CAD build for the part. Positions are in the model's coordinates, mm. A direction names the side the tool comes from. Round coordinates to 2 decimals unless told otherwise and drop trailing zeros. Loops run counter-clockwise (first coordinate to the right, second up) from the corner with the lowest first, then second, coordinate; pieces in that order, holes last.
Autodesk Inventor part; units mm, degrees
ref_plane "Work Plane1" through (25, 0, 0) normal (1, 0, 0) x (0, 1, 0)
ref_plane "XZ Plane" through (0, 0, 0) normal (0, 1, 0) x (-1, 0, 0)
ref_plane "XY Plane" through (0, 0, 0) normal (0, 0, 1) x (1, 0, 0)
ref_plane "Work Plane1" through (25, 0, 0) normal (1, 0, 0) x (0, 1, 0)
sketch "Sketch1" plane through (0, 0, 0) normal (0, 0, 1) x (1, 0, 0)
  line L0 (0, 0) -> (50, 0)
  line L1 (50, 0) -> (50, 40)
  line L2 (50, 40) -> (0, 40)
  line L3 (0, 40) -> (0, 0)
  dimension "d0" = 50
  dimension "d1" = 40
extrude "Extrusion1" add sketch "Sketch1" along normal blind 30
sketch "Sketch3" plane through (50, 0, 0) normal (1, 0, 0) x (0, 0, -1)
  line L0 (0, 0) -> (-8, 40)
  line L1 (0, 40) -> (-30, 40)
  line L2 (0, 0) -> (40.7922, 0) construction
  arc A0 (0, 40) -> (-8, 40) centre (-4, 20) ccw
  line L3 (0, 0) -> (0, 40)
  line L4 (0, 40) -> (0, 0)
  dimension "d7" = 101.31
extrude "Extrusion3" cut sketch "Sketch3" against normal through all contours L0 L1 L3
sketch "Sketch4" plane through (0, 0, 30) normal (0, 0, 1) x (1, 0, 0)
  line L0 (0, 0) -> (50, 0) construction
  line L1 (25, 0) -> (25, 40) construction
  line L2 (50, 40) -> (0, 40) construction
  line L3 (0, 40) -> (0, 0) construction
  line L4 (0, 20) -> (50, 20) construction
  line L5 (50, 0) -> (50, 40) construction
  line L6 (17.5, 10) -> (17.5, 30)
  line L7 (32.5, 10) -> (32.5, 30)
  line L8 (12.5, 10) -> (12.5, 30)
  line L9 (37.5, 10) -> (37.5, 30)
  line L10 (12.5, 10) -> (17.5, 10)
  line L11 (32.5, 10) -> (37.5, 10)
  line L12 (12.5, 30) -> (17.5, 30)
  line L13 (32.5, 30) -> (37.5, 30)
  dimension "d12" = 7.5
  dimension "d13" = 7.5
  dimension "d14" = 5
  dimension "d15" = 20
  dimension "d16" = 5
  dimension "d17" = 20
  dimension "d18" = 10
  dimension "d19" = 10
extrude "Extrusion4" add sketch "Sketch4" along normal blind 22.5
fillet "Fillet1" radius 10 4 edges at (15, 10, 52.5) (15, 30, 52.5) (35, 10, 52.5) (35, 30, 52.5)
sketch "Sketch5" plane through (37.5, 10, 30) normal (1, 0, 0) x (0, 0, -1)
  arc A0 (-12.5, 20) -> (-12.5, 0) centre (-12.5, 10) ccw
  line L0 (-12.5, 0) -> (-12.5, 20) construction
  circle A1 centre (-12.5, 10) radius 3.75
  point P0 (30, -10)
  dimension "d23" = 7.5
extrude "Extrusion5" cut sketch "Sketch5" against normal through all
sketch "Sketch6" plane through (25, 0, 0) normal (1, 0, 0) x (0, 1, 0)
  line L0 (40, 8) -> (40, 30)
  line L1 (0, 0) -> (40, 8)
  line L2 (40, 8) -> (40, 13.0991)
  line L3 (40, 13.0991) -> (0, 5.099)
  line L4 (0, 5.099) -> (0, 0)
  dimension "d27" = 5
extrude "Extrusion6" add sketch "Sketch6" along normal mid plane 90
sketch "Sketch7" plane through (50, 0, 5.099) normal (0, -0.1961173, 0.9805804) x (1, 0, 0)
  circle A0 centre (12.5, 10) radius 2.5
  circle A1 centre (12.5, 30.7922) radius 2.5
  line L0 (20, 40.7922) -> (20, 0)
  line L1 (0, 0) -> (20, 0)
  line L2 (0, 40.7922) -> (20, 40.7922)
  point P0 (-50, -1)
  dimension "d30" = 5
  dimension "d31" = 5
  dimension "d32" = 7.5
  dimension "d33" = 7.5
  dimension "d34" = 10
  dimension "d35" = 10
extrude "Extrusion7" cut sketch "Sketch7" against normal through all
mirror "Mirror1" about plane through (25, 0, 0) normal (1, 0, 0) of "Extrusion7"
chamfer "Chamfer1" distance 3 angle 45 4 edges at (70, 0, 2.5495) (70, 40, 10.5496) (-20, 0, 2.5495) (-20, 40, 10.5496)
properties part number "Base"
Item 1: Cut at D-D, the plane y = 5. Give the cut face in (x, z), plus the area to 3 significant figures.
Answers follow:
outline: (-20, 1) - (70, 1) - (70, 6.1) - (50, 6.1) - (50, 30) - (0, 30) - (0, 6.1) - (-20, 6.1) - close
area: 1,650 mm2
Item 2: Cut at A-A, the plane z = 33.5. Give the cut face in (x, y).
Answers follow:
outline: (12.5, 10) - (17.5, 10) - (17.5, 30) - (12.5, 30) - close; (32.5, 10) - (37.5, 10) - (37.5, 30) - (32.5, 30) - close
Item 3: 3-axis set-ups, long thin cutter, end or side, ignore diameter. For faces 1 (the flat face through (15, 30, 36)), 2 (the flat face through (15, 10, 36)), 3 (the flat face through (-10.14, 20.28, 9.155)): which of +Z, -Z, +X, -X, +Y, -Y reach the whole face in a straight line?
Answers follow:
face 1: +Z, +X, -X, +Y
face 2: +Z, +X, -X, -Y
face 3: +Z, -X, -Y
Item 4: Two-plate mould, pull along X, no slides. Class faces 4 (the flat face through (50, 20, 20)), 5 (the cylindrical face through (-14.81, 11.23, 4.83)), 6 (the flat face through (35, 30, 36)): released by +X, released by -X, zero draft, split by the parting line, or undercut.
Answers follow:
face 4: released by +X
face 5: undercut
face 6: zero draft
Item 5: Cut at C-C, the plane y = 18. Give the cut face in (x, z).
Answers follow:
outline: (-20, 3.6) - (70, 3.6) - (70, 8.7) - (50, 8.7) - (50, 30) - (37.5, 30) - (37.5, 39.33) - (32.5, 39.33) - (32.5, 30) - (17.5, 30) - (17.5, 39.33) - (12.5, 39.33) - (12.5, 30) - (0, 30) - (0, 8.7) - (-20, 8.7) - close; (12.5, 45.67) - (17.5, 45.67) - (17.5, 52.3) - (12.5, 52.3) - close; (32.5, 45.67) - (37.5, 45.67) - (37.5, 52.3) - (32.5, 52.3) - close
Item 6: Flat gauge pins, fed straight in: P1, Ø4, axis at x = -5, y = 15.5, coming from the +Z side; P2, Ø10, axis at y = 20, z = 42.5, coming from the +X side; P3, Ø12, axis at y = 20, z = 42.5, coming from the -X side. Where does each tip first touch, or does it go through?
Answers follow:
P1: stops at z = 8.6
P2: stops at x = 37.5
P3: stops at x = 12.5
Item 7: Probe line 1 (X direction, y = 12, z = 42.5); line 2 (Y direction, x = 14.7, z = 42.5); line 3 (Z direction, x = 25, y = 25.5). List the from-to ranges inside material, lowest first.
Answers follow:
line 1: x = 12.5 to 17.5, 32.5 to 37.5
line 2: y = 10 to 16.25, 23.75 to 30
line 3: z = 5.1 to 30
